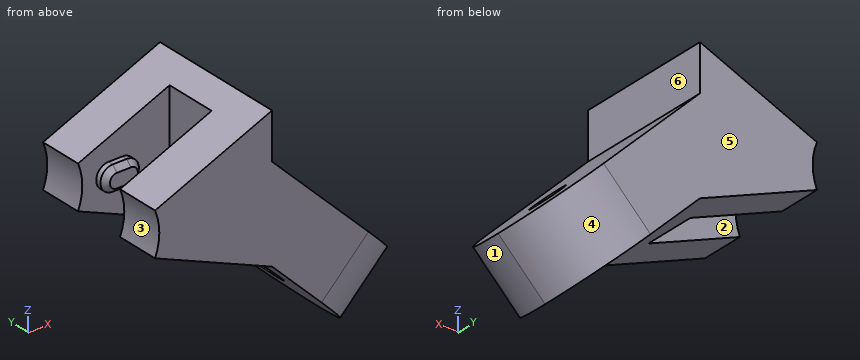
from build123d import *

# Parameters (mm, degrees)
AUFSATZ_LINEAR_AUSTRAGEN1_DEPTH             = 4
SCHNITT_LINEAR_AUSTRAGEN1_DEPTH             = 12.191730608
SCHNITT_LINEAR_AUSTRAGEN1_DEPTH_BACK        = 12.191730608
SKIZZE2_W                                   = 8.2
SKIZZE2_H                                   = 3
AUFSATZ_LINEAR_AUSTRAGEN2_DEPTH             = 0.6
FASE1_SIZE                                  = 0.3
FASE1_OF_SPIEGELN1_SIZE                     = 0.3
AUFSATZ_LINEAR_AUSTRAGEN5_REACH             = 13.192
AUFSATZ_LINEAR_AUSTRAGEN5_DIRECTION_2_REACH = 13.192
VERRUNDUNG2_R                               = 4
SKIZZE15_R                                  = 1
SCHNITT_LINEAR_AUSTRAGEN2_DEPTH             = 21.051946243


with BuildPart() as part:
    # Skizze1 → Aufsatz-Linear austragen1 (new, symmetric)
    with BuildSketch(Plane(origin=(0, 0, 0), x_dir=(1, 0, 0), z_dir=(0, 1, 0))):
        with BuildLine():
            Line((2.956414504, 1.224586984), (9.656854249, 4))
            Line((9.656854249, 4), (9.656854249, -4))
            Line((9.656854249, -4), (2.956414504, -1.224586984))
            ThreePointArc((2.956414504, -1.224586984), (3.2, 0), (2.956414504, 1.224586984))
        make_face()
    extrude(amount=AUFSATZ_LINEAR_AUSTRAGEN1_DEPTH, both=True)

    # Skizze2 → Schnitt-Linear austragen1 (cut, two sides: drawn at the far end of the back side and taken through both)
    with BuildSketch(Plane.XY.offset(-SCHNITT_LINEAR_AUSTRAGEN1_DEPTH_BACK)):
        with Locations((4.1, 0)):
            Rectangle(SKIZZE2_W, SKIZZE2_H)
    extrude(amount=SCHNITT_LINEAR_AUSTRAGEN1_DEPTH + SCHNITT_LINEAR_AUSTRAGEN1_DEPTH_BACK, mode=Mode.SUBTRACT)

    # Skizze7 → Aufsatz-Linear austragen2 (add)
    with BuildSketch(Plane.XZ.offset(-1.5)):
        with BuildLine():
            Line((4.7, 0.7), (5.5, 0.7))
            ThreePointArc((5.5, 0.7), (6.2, 0), (5.5, -0.7))
            Line((5.5, -0.7), (4.7, -0.7))
            ThreePointArc((4.7, -0.7), (4, 0), (4.7, 0.7))
        make_face()
    aufsatz_linear_austragen2 = extrude(amount=AUFSATZ_LINEAR_AUSTRAGEN2_DEPTH)

    # Fase1
    fase1_edges = [part.edges().sort_by_distance(p)[0] for p in [
        (4, 0.9, 0),
        (5.1, 0.9, -0.7),
        (6.2, 0.9, 0),
        (5.1, 0.9, 0.7),
    ]]
    chamfer(fase1_edges, length=FASE1_SIZE)

    # Spiegeln1: Aufsatz-Linear austragen2 across plane
    add(aufsatz_linear_austragen2.mirror(Plane.ZX))

    # Fase1 of Spiegeln1
    fase1_of_spiegeln1_edges = [part.edges().sort_by_distance(p)[0] for p in [
        (4, -0.9, 0),
        (5.1, -0.9, -0.7),
        (6.2, -0.9, 0),
        (5.1, -0.9, 0.7),
    ]]
    chamfer(fase1_of_spiegeln1_edges, length=FASE1_OF_SPIEGELN1_SIZE)

    # Aufsatz-Linear austragen5: up to this face of the body (flat: up to its plane)
    aufsatz_linear_austragen5_end = Plane(part.part.faces().sort_by_distance((6.944416323, 4, 0))[0])
    # Skizze13 → Aufsatz-Linear austragen5 (add, up to the picked face)
    with BuildSketch(Plane(origin=(0, 0, 0), x_dir=(1, 0, 0), z_dir=(0, 1, 0)), mode=Mode.PRIVATE) as aufsatz_linear_austragen5_sk1:
        Polygon((9.656854249, 4), (15.313708499, 9.656854249), (18.000714267, 6.969848481), (9.656854249, -1.374011537), align=None)
    aufsatz_linear_austragen5_tool1 = split(extrude(aufsatz_linear_austragen5_sk1.sketch, amount=AUFSATZ_LINEAR_AUSTRAGEN5_REACH, mode=Mode.PRIVATE), bisect_by=aufsatz_linear_austragen5_end, keep=Keep.BOTH, mode=Mode.PRIVATE)
    add(aufsatz_linear_austragen5_tool1.solids().sort_by(Axis((13.200007, 0, -4.684251), (0, 1, 0)))[0])

    # Aufsatz-Linear austragen5 direction 2: up to this face of the body (flat: up to its plane)
    aufsatz_linear_austragen5_direction_2_end = Plane(part.part.faces().sort_by_distance((6.944416323, -4, 0))[0])
    # Skizze13 → Aufsatz-Linear austragen5 direction 2 (add, up to the picked face)
    with BuildSketch(Plane(origin=(0, 0, 0), x_dir=(1, 0, 0), z_dir=(0, 1, 0)), mode=Mode.PRIVATE) as aufsatz_linear_austragen5_direction_2_sk1:
        Polygon((9.656854249, 4), (15.313708499, 9.656854249), (18.000714267, 6.969848481), (9.656854249, -1.374011537), align=None)
    aufsatz_linear_austragen5_direction_2_tool1 = split(extrude(aufsatz_linear_austragen5_direction_2_sk1.sketch, amount=-AUFSATZ_LINEAR_AUSTRAGEN5_DIRECTION_2_REACH, mode=Mode.PRIVATE), bisect_by=aufsatz_linear_austragen5_direction_2_end, keep=Keep.BOTH, mode=Mode.PRIVATE)
    add(aufsatz_linear_austragen5_direction_2_tool1.solids().sort_by(Axis((13.200007, 0, -4.684251), (0, -1, 0)))[0])

    # Verrundung2
    verrundung2_edges = [part.edges().sort_by_distance(p)[0] for p in [
        (16.657211383, 4, -8.313351365),
        (16.657211383, -4, -8.313351365),
    ]]
    fillet(verrundung2_edges, radius=VERRUNDUNG2_R - 0.0001)  # a hair under: the kernel refuses the full size

    # Skizze15 → Schnitt-Linear austragen2 (cut, through all)
    with BuildSketch(Plane(origin=(5.515432893, 0, 5.515432893), x_dir=(0.707106781186546, 0, -0.707106781186549), z_dir=(0.707106781186549, 0, 0.707106781186546))):
        with Locations((13.656854249, 0)):
            Circle(SKIZZE15_R)
    extrude(amount=-SCHNITT_LINEAR_AUSTRAGEN2_DEPTH, mode=Mode.SUBTRACT)


solid = part.part
Geometry: final body of the model. Coordinates: model frame, mm. Face numbers are marked on the shaded views. A direction names the side the tool comes from. Coordinates: 2 decimals unless noted, no trailing zeros. Loops run counter-clockwise (first coordinate to the right, second up) from the corner with the lowest first, then second, coordinate; pieces in that order, holes last. Notation, with made-up numbers: (11, 85.25) - (69, 85.25) arc R17 cw to (69, 115.25) - close; hole circle Ø1 at (33, 60.5). An arc over 180 degrees is marked (long way). One line per question, with ' | ' between items. Start each with the question number.
(1) Cut plane B-B on z = 0. Output: boundary loops of the cut face in (x, y), and give its area (3 significant figures).
(2) Draft query along Y for the marked faces 1, 2, 3 and 4. Return one class per face: +Y half, -Y half, draft (parallel to the pull), parting line (faces both ways), or undercut.
(3) Ray query, L1, parallel to X at y = -0.5, z = -5.5; L2, parallel to Y at x = 14, z = -4.5; L3, parallel to X at y = -0.75, z = -5.75. Return the intervals inside material, ascending. Write a range as from..to.
(4) First-contact query: pin 1 (3 mm diameter, centred on x = 10, y = 0, fed in from -Z); pin 2 (2 mm diameter, centred on y = 0, z = 3, fed in from +X). Flat tips, straight axial feed; report the tip coordinate or a pass-through.
(5) Reachability of the marked faces 5 and 6 from +Z, -Z, +X, -X, +Y, -Y: full face, straight path, thin tool, end or side. Return the list, or none.
(6) Cut plane C-C on x = 10.75. Output: boundary loops of the cut face in (y, z).
(7) Cut plane D-D on y = 3. Output: boundary loops of the cut face in (x, z), and give its area (3 significant figures).
(8) Cut plane A-A on y = -2. Output: boundary loops of the cut face in (x, z), and give its area (3 significant figures).
Here are the results:
1) outline: (3.2, -4) - (11.03, -4) - (11.03, 4) - (3.2, 4) - (3.2, 1.5) - (4, 1.5) - (4, 1.2) - (4.3, 0.9) - (5.9, 0.9) - (6.2, 1.2) - (6.2, 1.5) - (8.2, 1.5) - (8.2, -1.5) - (6.2, -1.5) - (6.2, -1.2) - (5.9, -0.9) - (4.3, -0.9) - (4, -1.2) - (4, -1.5) - (3.2, -1.5) - close | area: 50.1 mm²
2) face 1: -Y half | face 2: undercut | face 3: draft | face 4: +Y half
3) L1: 11.16..12.59, 15.04..16.53 | L2: -4..-0.82, 0.82..4 | L3: 11.41..12.63, 14.5..16.78
4) pin 1: z = -5.84 | pin 2: x = 9.66
5) face 5: +Z, -Z, +X, -X, +Y | face 6: +Z, +X, +Y, -Y
6) outline: (-4, -5.09) - (4, -5.09) - (4, 0.28) - (-4, 0.28) - close
7) outline: (2.96, -1.22) - (9.66, -4) - (14.36, -8.7) - (17.04, -6.01) - (9.66, 1.37) - (9.66, 4) - (2.96, 1.22) arc R3.2 cw to start | area: 67.1 mm²
8) outline: (2.96, -1.22) - (9.66, -4) - (14.93, -9.28) - (17.62, -6.59) - (9.66, 1.37) - (9.66, 4) - (2.96, 1.22) arc R3.2 cw to start | area: 70.2 mm²
